Verification items for the finished model (mm, model axes). A direction names the side the tool comes from. Give positions to 0.01 mm unless a question says otherwise; leave off trailing zeros. Write each loop counter-clockwise with the first axis right and the second up, starting at its lowest first coordinate (ties: lowest second). Pieces come first, ordered by that corner, then holes. Notation, with made-up numbers: M 60.25,65 L 109.25,65 A20 ccw 109.25,76 Z; hole C 52.5,32.5 d1. An arc over 180 degrees is marked long. Write item = value, one per line.
from build123d import *

# Parameters (mm, degrees)
SKETCH1_W      = 50
SKETCH1_H      = 33
EXTRUDE1_DEPTH = 5


with BuildPart() as part:
    # Sketch1 → Extrude1 (new body)
    with BuildSketch(Plane(origin=(0, 0, 0), x_dir=(0, 0, -1), z_dir=(1, 0, 0))):
        Rectangle(SKETCH1_W, SKETCH1_H)
        with BuildLine():
            Line((-20, 4.25), (-10, 4.25))
            ThreePointArc((-10, 4.25), (-7.25, 1.5), (-10, -1.25))
            Line((-10, -1.25), (-20, -1.25))
            ThreePointArc((-20, -1.25), (-22.75, 1.5), (-20, 4.25))
        make_face(mode=Mode.SUBTRACT)
    extrude(amount=EXTRUDE1_DEPTH)


solid = part.part
1) Draft check along Y on faces 3 (the cylindrical face through (2.46, 1.56, 7.25)), 4 (the flat face through (5, 0, 0)), 5 (the flat face through (2, -16.5, 0)). Enter one of: +Y half, -Y half, draft (parallel to the pull), parting line (faces both ways), or undercut.
From the geometry:
face_3 = undercut
face_4 = draft
face_5 = -Y half
2) Tool access check on faces 1 (the flat face through (0, 0, 0)), 2 (the cylindrical face through (2.46, 1.44, 22.75)). Record the directions out of +Z, -Z, +X, -X, +Y, -Y that give a thin tool (end or side, any length) a straight path to the whole face; none if there is none.
From the geometry:
face_1 = +Z, -Z, -X, +Y, -Y
face_2 = +X, -X
3) Cross-section at B-B on y = 1.5. Record the boundary of the cut face in (x, z), plus the area to 4 significant figures.
From the geometry:
outline = M 0,-25 L 5,-25 L 5,7.25 L 0,7.25 Z; M 0,22.75 L 5,22.75 L 5,25 L 0,25 Z
area = 172.5 mm^2
4) Cross-section at A-A on x = 0.7. Record the boundary of the cut face in (y, z).
From the geometry:
outline = M -16.5,-25 L 16.5,-25 L 16.5,25 L -16.5,25 Z; hole M -1.25,10 A2.75 ccw 4.25,10 L 4.25,20 A2.75 ccw -1.25,20 Z
5) Material ranges on probe 1 along Z at (x, y) = (0.95, 3.5); probe 2 along Y at (x, z) = (2.85, 21.5); probe 3 along Z at (x, y) = (3.55, 3), recorded low to high. Write a range as from..to.
From the geometry:
probe_1 = -25..8.11, 21.89..25
probe_2 = -16.5..-0.8, 3.8..16.5
probe_3 = -25..7.7, 22.3..25
6) Depth check by flat-ended pin: P1, Ø8, axis at y = -0.5, z = -8.5, coming from the -X side. Enter the tip coordinate at first touch or a pass-through.
From the geometry:
P1 = 0
